```python
from build123d import *

# Parameters (mm, degrees)
BOSS_EXTRUDE1_DEPTH     = 139.7
SKETCH3_W               = 127
SKETCH3_H               = 63.5
SKETCH3_R               = 1.5875
CUT_EXTRUDE1_DEPTH      = 10.525
CUT_EXTRUDE1_DEPTH_BACK = 4.175


with BuildPart() as part:
    # Sketch2 → Boss-Extrude1 (new body)
    with BuildSketch(Plane(origin=(0, 0, 0), x_dir=(1, 0, 0), z_dir=(0, 1, 0))):
        Polygon((0, 0), (0, 12.7), (3.175, 12.7), (3.175, 3.175), (123.825, 3.175), (123.825, 12.7), (127, 12.7), (127, 0), align=None)
    extrude(amount=BOSS_EXTRUDE1_DEPTH)

    # Sketch3 → Cut-Extrude1 (cut, two sides)
    with BuildSketch(Plane(origin=(0, 0, -3.175), x_dir=(-1, 0, 0), z_dir=(0, 0, -1))) as cut_extrude1_sk:
        with Locations((-63.5, 31.75)):
            Rectangle(SKETCH3_W, SKETCH3_H)
        with Locations((-97.536, 107.95)):
            Circle(SKETCH3_R)
        with Locations((-29.464, 107.95)):
            Circle(SKETCH3_R)
        with Locations((-29.464, 91.948)):
            Circle(SKETCH3_R)
        with Locations((-97.536, 91.948)):
            Circle(SKETCH3_R)
    extrude(amount=CUT_EXTRUDE1_DEPTH, mode=Mode.SUBTRACT)
    extrude(cut_extrude1_sk.sketch, amount=-CUT_EXTRUDE1_DEPTH_BACK, mode=Mode.SUBTRACT)


solid = part.part
```
Part model, mm, in its own coordinate system. A direction names the side the tool comes from. Round coordinates to 2 decimals unless told otherwise and drop trailing zeros. Order: outer loops, then holes, each group sorted by start corner. A loop starts at its lowest first (then second) coordinate and runs counter-clockwise, first axis right, second up. Notation, with made-up numbers: M 69.5,57 L 84.5,57 A19 cw 84.5,79 Z; hole C 58,-30.75 d6. An arc over 180 degrees is marked long. Put each result on its own line as item: value. Start each with the question number.
1. Slice it at D-D on y = 117.5. List the corners of the cut face in (x, z) (3 decimals).
2. Drill centre lines: probe 1 along X at (y, z) = (107.95, -2.05); probe 2 along X at (y, z) = (102, -6.25) (3 decimals); probe 3 along Z at (x, y) = (6.5, 68) (3 decimals). Where is each one in solid material? Low to high. Write a range as [from, to].
3. Slice it at B-B on z = -8.25. List the corners of the cut face in (x, y) (3 decimals), then the cut area to 3 significant figures.
4. Slice it at A-A on y = 107.95. List the corners of the cut face in (x, z) (1 decimal).
5. Two-plate mould, pull along X, no slides. Class faces 3 (the face through (0, 101, -6)), 4 (the face through (123.825, 101, -8)), 5 (the face through (64, 101, 0)), 6 (the face through (29.8, 106.4, -1.6)): +X half, -X half, draft (parallel to the pull), parting line (faces both ways), or undercut.
6. Tool access for faces 1 (the face through (3.175, 101, -8)), 2 (the face through (64, 139.7, -3)): list every direction of +Z, -Z, +X, -X, +Y, -Y with a clear straight run to the whole face (end or side of a thin tool).
7. Drop flat-ended pins along their axis: pin 1 (5 mm diameter, centred on x = 29.464, y = 91.948, fed in from -Z) (3 decimals); pin 2 (2.5 mm diameter, centred on x = 29.464, y = 107.95, fed in from +Z) (3 decimals). Give the stop position or say it passes through.
8. Slice it at C-C on x = 29.5. List the corners of the cut face in (y, z) (3 decimals).
Findings:
1. outline: M 0,-12.7 L 3.175,-12.7 L 3.175,-3.175 L 123.825,-3.175 L 123.825,-12.7 L 127,-12.7 L 127,0 L 0,0 Z
2. probe 1: [0, 27.88], [31.05, 95.95], [99.12, 127]
2. probe 2: [0, 3.175], [123.825, 127]
2. probe 3: [-3.175, 0]
3. outline: M 0,63.5 L 3.175,63.5 L 3.175,139.7 L 0,139.7 Z; M 123.825,63.5 L 127,63.5 L 127,139.7 L 123.825,139.7 Z
3. area: 484 mm2
4. outline: M 0,-12.7 L 3.2,-12.7 L 3.2,-3.2 L 27.9,-3.2 L 27.9,0 L 0,0 Z; M 31.1,-3.2 L 95.9,-3.2 L 95.9,0 L 31.1,0 Z; M 99.1,-3.2 L 123.8,-3.2 L 123.8,-12.7 L 127,-12.7 L 127,0 L 99.1,0 Z
5. face 3: -X half
5. face 4: undercut
5. face 5: draft
5. face 6: undercut
6. face 1: -Z, +Y, -Y
6. face 2: +Z, -Z, +X, -X, +Y
7. pin 1: z = -3.175
7. pin 2: through
8. outline: M 63.5,-3.175 L 90.361,-3.175 L 90.361,0 L 63.5,0 Z; M 93.535,-3.175 L 106.363,-3.175 L 106.363,0 L 93.535,0 Z; M 109.537,-3.175 L 139.7,-3.175 L 139.7,0 L 109.537,0 Z
